```python
from build123d import *

# Parameters (mm, degrees)
DODANIE_WYCI_GNI_CIE1_DEPTH = 1.5
ZAOKR_GLENIE1_R             = 2


with BuildPart() as part:
    # Szkic1 → Dodanie-wyciągnięcie1 (new body)
    with BuildSketch(Plane.XY):
        Polygon((-10.705397727, 7.837073864), (8.494602273, 7.837073864), (8.494602273, -0.462926136), (6.294602273, -2.562926136), (6.294602273, -8.062926136), (-8.505397727, -8.062926136), (-8.505397727, -2.562926136), (-10.705397727, -0.462926136), align=None)
    extrude(amount=DODANIE_WYCI_GNI_CIE1_DEPTH)

    # Zaokrąglenie1
    zaokr_glenie1_edges = [part.edges().sort_by_distance(p)[0] for p in [
        (-10.705397727, 7.837073864, 0.75),
        (8.494602273, 7.837073864, 0.75),
        (6.294602273, -8.062926136, 0.75),
        (-8.505397727, -8.062926136, 0.75),
    ]]
    fillet(zaokr_glenie1_edges, radius=ZAOKR_GLENIE1_R)


solid = part.part
```
Read the model definition and answer for the solid it produces. Units are mm, in the model's axes. A direction names the side the tool comes from. Round coordinates to 2 decimals unless told otherwise and drop trailing zeros. Loops run counter-clockwise (first coordinate to the right, second up) from the corner with the lowest first, then second, coordinate; pieces in that order, holes last. Notation, with made-up numbers: (-19, 52.25) -> (18, 52.25) arc R13 cw to (18, 64.25) -> close; hole circle Ø7 at (49.5, -24). An arc over 180 degrees is marked (long way). One line per item, written item: value.
1) Consider L1, parallel to X at y = -2.75, z = 0.6; L2, parallel to Y at x = -9.25, z = 0.6; L3, parallel to Y at x = 5.5, z = 0.45. Determine where each line is inside the solid, lowest interval first. Write a range as [from, to].
Answer list:
L1: x = [-8.51, 6.29]
L2: y = [-1.85, 7.76]
L3: y = [-7.66, 7.84]
2) For faces 1 (the face through (6.295, -4, 1)), 2 (the face through (-10.1, 7.27, 0.76)), 3 (the face through (-8.505, -4, 1)), determine the directions among +Z, -Z, +X, -X, +Y, -Y from which every point of the face is accessible in a straight line to the end or side of a thin tool.
Answer list:
face 1: +Z, -Z, +X, -Y
face 2: +Z, -Z, -X, +Y
face 3: +Z, -Z, -X, -Y
3) A cutting plane is placed at B-B (y = -4.5). Determine the outline of the cut face in (x, z), and give its area (3 significant figures).
Answer list:
outline: (-8.51, 0) -> (6.29, 0) -> (6.29, 1.5) -> (-8.51, 1.5) -> close
area: 22.2 mm²
4) A flat-ended cylindrical pin translates along its axis: P1, Ø1, axis at x = -4, y = -3, coming from the -Z side. Find the tip coordinate at first contact, or state that the pin passes through.
Answer list:
P1: stops at z = 0
5) A cutting plane is placed at A-A (z = 0.9). Determine the outline of the cut face in (x, y).
Answer list:
outline: (-10.71, -0.46) -> (-8.51, -2.56) -> (-8.51, -6.06) arc R2 ccw to (-6.51, -8.06) -> (4.29, -8.06) arc R2 ccw to (6.29, -6.06) -> (6.29, -2.56) -> (8.49, -0.46) -> (8.49, 5.84) arc R2 ccw to (6.49, 7.84) -> (-8.71, 7.84) arc R2 ccw to (-10.71, 5.84) -> close
6) A cutting plane is placed at C-C (x = 7). Determine the outline of the cut face in (y, z), and give its area (3 significant figures).
Answer list:
outline: (-1.89, 0) -> (7.77, 0) -> (7.77, 1.5) -> (-1.89, 1.5) -> close
area: 14.5 mm²
